The listing builds one solid part. Answer for the finished solid, in the listing's coordinates (mm). A direction names the side the tool comes from. Round coordinates to 2 decimals unless told otherwise and drop trailing zeros. Order: outer loops, then holes, each group sorted by start corner. A loop starts at its lowest first (then second) coordinate and runs counter-clockwise, first axis right, second up. Notation, with made-up numbers: M 14.5,2.5 L 22.5,2.5 A19 cw 22.5,25.5 Z; hole C 75.25,37.25 d8. An arc over 180 degrees is marked long. Put each result on its own line as item: value. Start each with the question number.
1. Consider line 1 (X direction, y = 2.5, z = 6); line 2 (Z direction, x = 43.5, y = 5.08) (3 decimals); line 3 (X direction, y = 20.75, z = 3.5). Determine where each line is inside the solid, lowest interval first.
2. The mould has two halves that part along X. Classify faces 1 (the face through (1.582, 7, 3)), 2 (the face through (23.575, 24.577, 3.131)), 3 (the face through (43.422, 6.766, 3.396)), 4 (the face through (4.757, 8, 3)): +X half, -X half, draft (parallel to the pull), parting line (faces both ways), or undercut.
3. The part is cut by section A-A (y = 11.25). Give the vertices of the cut face in (x, z).
4. The part is cut by section D-D (y = 23.5). Give the vertices of the cut face in (x, z).
5. Each of these flat-tipped pins is pushed along its axis until it touches: pin 1 Ø1.7 at (x, z) = (5, 3) entering from +Y; pin 2 Ø3 at (x, z) = (38.5, 4.5) entering from -Y; pin 3 Ø2.5 at (y, z) = (5.08, 3.175) entering from +X; pin 4 Ø2 at (x, z) = (33.5, 2.5) entering from -Y. Where does it stop, or does it pass through?
6. Which of the six approach directions +Z, -Z, +X, -X, +Y, -Y give full straight-line access (tool end or side, diameter ignored) to faces 5 (the face through (42, 14.521, 3)), 6 (the face through (22, 25, 6.35)), 7 (the face through (4, 14.521, 3)), 8 (the face through (8, 12.38, 3))?
7. The part is cut by section C-C (z = 4). Give the vertices of the cut face in (x, y).
8. The part is cut by section B-B (y = 5.08). Give the vertices of the cut face in (x, z) (3 decimals).
from build123d import *

# Parameters (mm, degrees)
BOSS_EXTRUDE1_DEPTH     = 6.35
CUT_EXTRUDE1_DEPTH      = 53.418642591
CUT_EXTRUDE1_DEPTH_BACK = 53.418642591
SKETCH2_R               = 1.7


with BuildPart() as part:
    # Sketch1 → Boss-Extrude1 (new body)
    with BuildSketch(Plane.XY):
        with BuildLine():
            Line((39.411995156, 14.521042354), (45.031969649, 14.521042354))
            Line((45.031969649, 14.521042354), (45.031969649, 0))
            Line((45.031969649, 0), (41.856969649, 0))
            Line((41.856969649, 0), (41.856969649, 12.38))
            Line((41.856969649, 12.38), (35.506969649, 12.38))
            ThreePointArc((35.506969649, 12.38), (23.306969665, 24.579999984), (11.106969681, 12.38))
            Line((11.106969681, 12.38), (4.756969681, 12.38))
            Line((4.756969681, 12.38), (4.756969681, 0))
            Line((4.756969681, 0), (1.581969681, 0))
            Line((1.581969681, 0), (1.581969681, 14.521042354))
            Line((1.581969681, 14.521042354), (7.201944173, 14.521042354))
            ThreePointArc((7.201944173, 14.521042354), (23.306969665, 28.626719929), (39.411995156, 14.521042354))
        make_face()
    extrude(amount=BOSS_EXTRUDE1_DEPTH)

    # Sketch2 → Cut-Extrude1 (cut, two sides: drawn at the far end of the back side and taken through both)
    with BuildSketch(Plane(origin=(45.031969649, 0, 0), x_dir=(0, 0, -1), z_dir=(1, 0, 0)).offset(-CUT_EXTRUDE1_DEPTH_BACK)):
        with Locations((-3.175, 5.08)):
            Circle(SKETCH2_R)
    extrude(amount=CUT_EXTRUDE1_DEPTH + CUT_EXTRUDE1_DEPTH_BACK, mode=Mode.SUBTRACT)


solid = part.part
Resolved:
1. line 1: 1.58 to 4.76, 41.86 to 45.03
1. line 2: 0 to 1.475, 4.875 to 6.35
1. line 3: 9.38 to 14.43, 32.18 to 37.23
2. face 1: -X half
2. face 2: undercut
2. face 3: draft
2. face 4: undercut
3. outline: M 1.58,0 L 4.76,0 L 4.76,6.35 L 1.58,6.35 Z; M 41.86,0 L 45.03,0 L 45.03,6.35 L 41.86,6.35 Z
4. outline: M 11.46,0 L 18.29,0 L 18.29,6.35 L 11.46,6.35 Z; M 28.33,0 L 35.15,0 L 35.15,6.35 L 28.33,6.35 Z
5. pin 1: y = 14.52
5. pin 2: y = 12.38
5. pin 3: through
5. pin 4: y = 17.23
6. face 5: +Z, -Z, +X, +Y
6. face 6: +Z, +X, -X, +Y, -Y
6. face 7: +Z, -Z, -X, +Y
6. face 8: +Z, -Z, -Y
7. outline: M 1.58,0 L 4.76,0 L 4.76,3.59 L 1.58,3.59 Z; M 1.58,6.57 L 4.76,6.57 L 4.76,12.38 L 11.11,12.38 A12.2 cw 35.51,12.38 L 41.86,12.38 L 41.86,6.57 L 45.03,6.57 L 45.03,14.52 L 39.41,14.52 A16.25 ccw 7.2,14.52 L 1.58,14.52 Z; M 41.86,0 L 45.03,0 L 45.03,3.59 L 41.86,3.59 Z
8. outline: M 1.582,0 L 4.757,0 L 4.757,1.475 L 1.582,1.475 Z; M 1.582,4.875 L 4.757,4.875 L 4.757,6.35 L 1.582,6.35 Z; M 41.857,0 L 45.032,0 L 45.032,1.475 L 41.857,1.475 Z; M 41.857,4.875 L 45.032,4.875 L 45.032,6.35 L 41.857,6.35 Z
